Can you work these out from the model? Positions are in its coordinate system, mm. A direction names the side the tool comes from. Give positions to 0.01 mm unless a question says otherwise; leave off trailing zeros. Write each loop counter-clockwise with the first axis right and the second up, starting at its lowest first coordinate (ties: lowest second). Pieces come first, ordered by that corner, then holes.
1. On a 3-axis mill with a long thin cutter (end or side, diameter ignored), from which of +Z, -Z, +X, -X, +Y, -Y can I reach the whole of each face in a straight line? I mean faces 1 (the flat face through (3, 1.7, 4.9)), 2 (the flat face through (0, -4, 0)). Say none if no direction works.
2. If I drill on probe 1 along Y at (x, z) = (0, 5.75); probe 2 along Y at (x, z) = (-0.5, 3.5); probe 3 along Y at (x, z) = (-3.25, 1.75), over which ranges is the centre line in solid material (lowest first)?
3. Suppose I cut it at A-A (x = 0). Please give me the cut outline in (y, z), and give its area (3 significant figures).
4. I'm going to push flat-ended pins straight in: pin 1 (2.5 mm diameter, centred on x = 0, y = -6.35, fed in from +Z); pin 2 (4 mm diameter, centred on x = 4, z = 2.5, fed in from +Y); pin 3 (2 mm diameter, centred on y = -2.5, z = 2.5, fed in from -X); pin 4 (6 mm diameter, centred on y = -5.5, z = 2.5, fed in from +X). Where does each tip first touch, or does it pass through?
5. Suppose I cut it at D-D (y = -6.35). Please give me the cut outline in (x, z).
6. Thinking about a two-plate mould opening in Y: for faces 3 (the flat face through (0, -4, 10)), 4 (the flat face through (-3, -1.7, 4.9)), 5 (the flat face through (-3, 1.7, 4.9)), 6 (the cylindrical face through (-1.172, 8.923, 4.93)), which applies, pulls with the +Y half, pulls with the -Y half, needs draft (parallel to the pull), parting line crosses it, or undercut?
7. Suppose I cut it at C-C (x = -3.75). Please give me the cut outline in (y, z), and give its area (3 significant figures).
8. Suppose I cut it at B-B (z = 2.5). Please give me the cut outline in (x, y), and give its area (3 significant figures).
```python
from build123d import *

# Parameters (mm, degrees)
F0_R     = 9
F0_R_2   = 1.55
F1_DEPTH = 10


with BuildPart() as f1:
    # F0 (on Top) → F1 (new body)
    with BuildSketch(Plane.XY):
        Circle(F0_R)
        with Locations((0, -6.35)):
            Circle(F0_R_2, mode=Mode.SUBTRACT)
        with Locations((-6.35, 0)):
            Circle(F0_R_2, mode=Mode.SUBTRACT)
        Polygon((-3.983717, 0), (-1.991858, 3.45), (1.991858, 3.45), (3.983717, 0), (1.991858, -3.45), (-1.991858, -3.45), align=None, mode=Mode.SUBTRACT)
        with Locations((6.35, 0)):
            Circle(F0_R_2, mode=Mode.SUBTRACT)
        with Locations((0, 6.35)):
            Circle(F0_R_2, mode=Mode.SUBTRACT)
        with Locations((-6.35, 0)):
            Circle(F0_R_2)
        with Locations((6.35, 0)):
            Circle(F0_R_2)
    extrude(amount=F1_DEPTH)


solid = f1.part
```
Checks:
1. face 1: +Z, -Z
1. face 2: -Z, +X, -X, +Y, -Y
2. probe 1: y = -9 to -7.9, -4.8 to -3.45, 3.45 to 4.8, 7.9 to 9
2. probe 2: y = -8.99 to -7.82, -4.88 to -3.45, 3.45 to 4.88, 7.82 to 8.99
2. probe 3: y = -8.39 to -1.27, 1.27 to 8.39
3. outline: (-9, 0) - (-7.9, 0) - (-7.9, 10) - (-9, 10) - close; (-4.8, 0) - (-3.45, 0) - (-3.45, 10) - (-4.8, 10) - close; (3.45, 0) - (4.8, 0) - (4.8, 10) - (3.45, 10) - close; (7.9, 0) - (9, 0) - (9, 10) - (7.9, 10) - close
3. area: 49.0 mm2
4. pin 1: passes through
4. pin 2: stops at y = 8.77
4. pin 3: stops at x = -8.87
4. pin 4: stops at x = 8.65
5. outline: (-6.38, 0) - (-1.55, 0) - (-1.55, 10) - (-6.38, 10) - close; (1.55, 0) - (6.38, 0) - (6.38, 10) - (1.55, 10) - close
6. face 3: needs draft
6. face 4: undercut
6. face 5: undercut
6. face 6: parting line crosses it
7. outline: (-8.18, 0) - (-0.4, 0) - (-0.4, 10) - (-8.18, 10) - close; (0.4, 0) - (8.18, 0) - (8.18, 10) - (0.4, 10) - close
7. area: 156 mm2
8. outline: circle Ø18 at (0, 0); hole (-3.98, 0) - (-1.99, -3.45) - (1.99, -3.45) - (3.98, 0) - (1.99, 3.45) - (-1.99, 3.45) - close; hole circle Ø3.1 at (0, -6.35); hole circle Ø3.1 at (0, 6.35)
8. area: 198 mm2
